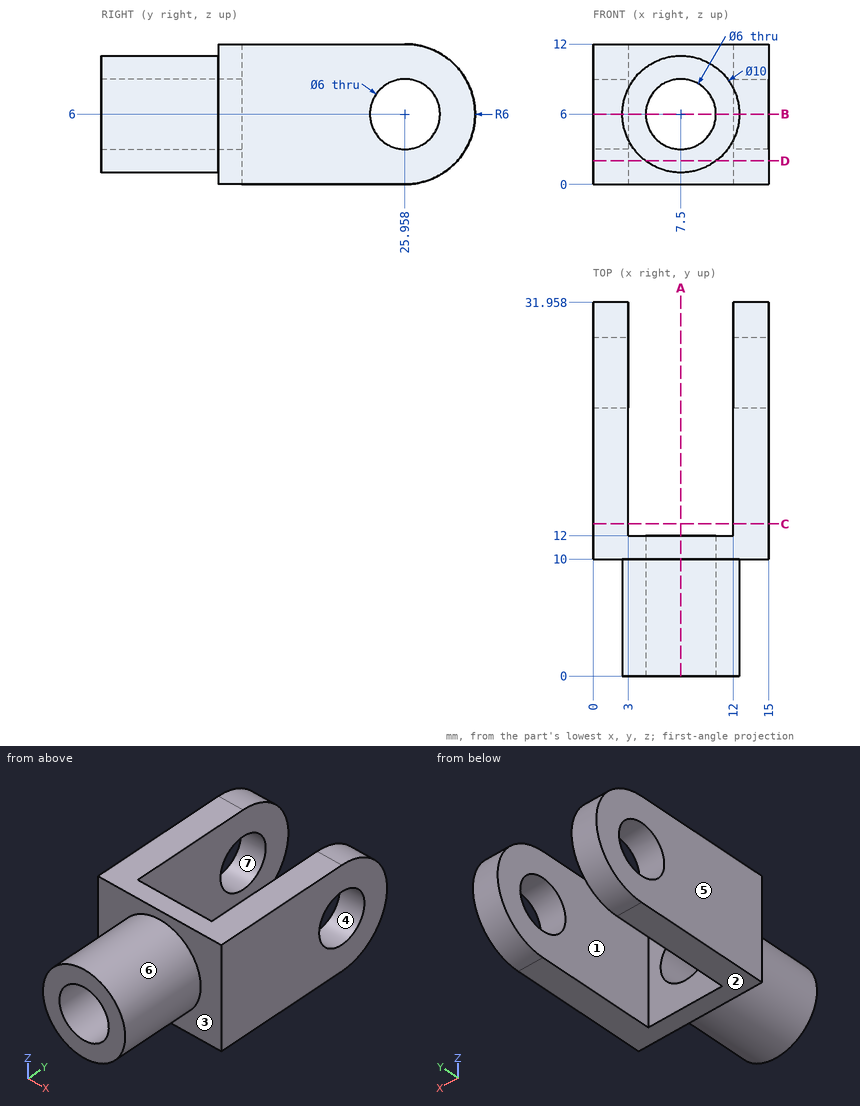
Check sheet for the drawn part. Datum: minimum x, y, z corner. Units: mm. A direction names the side the tool comes from. Round coordinates to 2 decimals unless told otherwise and drop trailing zeros. Write each loop counter-clockwise with the first axis right and the second up, starting at its lowest first coordinate (ties: lowest second). Pieces come first, ordered by that corner, then holes. Notation, with made-up numbers: (76.25, 38.25) -> (97.25, 38.25) arc R23 ccw to (97.25, 49.25) -> close; hole circle Ø1 at (-0.5, 0). An arc over 180 degrees is marked (long way). Put each result on its own line as item: value.
(1) Sectioned sample at B-B (z = 6). Enter the section's corners in (x, y).
Values found:
outline: (0, 10) -> (2.5, 10) -> (2.5, 0) -> (4.5, 0) -> (4.5, 12) -> (3, 12) -> (3, 22.96) -> (0, 22.96) -> close; (0, 28.96) -> (3, 28.96) -> (3, 31.96) -> (0, 31.96) -> close; (10.5, 0) -> (12.5, 0) -> (12.5, 10) -> (15, 10) -> (15, 22.96) -> (12, 22.96) -> (12, 12) -> (10.5, 12) -> close; (12, 28.96) -> (15, 28.96) -> (15, 31.96) -> (12, 31.96) -> close
(2) Sectioned sample at A-A (x = 7.5). Enter the section's corners in (y, z).
Values found:
outline: (0, 1) -> (10, 1) -> (10, 0) -> (12, 0) -> (12, 3) -> (0, 3) -> close; (0, 9) -> (12, 9) -> (12, 12) -> (10, 12) -> (10, 11) -> (0, 11) -> close
(3) Mould release check, pull along Z, two halves, no side actions. Record for the marked faces 4, 5, 6 and 7: released by +Z, released by -Z, zero draft, split by the parting line, or undercut.
Values found:
face 4: undercut
face 5: zero draft
face 6: split by the parting line
face 7: undercut
(4) Sectioned sample at D-D (z = 2). Enter the section's corners in (x, y).
Values found:
outline: (0, 10) -> (4.5, 10) -> (4.5, 0) -> (10.5, 0) -> (10.5, 10) -> (15, 10) -> (15, 30.43) -> (12, 30.43) -> (12, 12) -> (3, 12) -> (3, 30.43) -> (0, 30.43) -> close
(5) Material ranges on line 1 (X direction, y = 13, z = 0.75); line 2 (Y direction, x = 13.8, z = 6); line 3 (X direction, y = 4, z = 6), recorded low to high.
Values found:
line 1: x = 0 to 3, 12 to 15
line 2: y = 10 to 22.96, 28.96 to 31.96
line 3: x = 2.5 to 4.5, 10.5 to 12.5
(6) Tool access check on the marked faces 1, 2 and 3. Record the directions out of +Z, -Z, +X, -X, +Y, -Y that give a thin tool (end or side, any length) a straight path to the whole face; none if there is none.
Values found:
face 1: +Z, -Z, +Y
face 2: -Z, +X, -X, +Y, -Y
face 3: -Y
(7) Go/stop test with a flat-tipped pin: pin 1 Ø6 at (x, y) = (6, 5) entering from -Z. Record where the tip stops, or that it passes through.
Values found:
pin 1: stops at z = 1
(8) Sectioned sample at C-C (y = 13). Enter the section's corners in (x, z).
Values found:
outline: (0, 0) -> (3, 0) -> (3, 12) -> (0, 12) -> close; (12, 0) -> (15, 0) -> (15, 12) -> (12, 12) -> close
